from build123d import *

# Parameters (mm, degrees)
SKETCH1_W           = 100
SKETCH1_H           = 113.5
BOSS_EXTRUDE1_DEPTH = 8.5
CUT_EXTRUDE1_REACH  = 78.111
SKETCH2_W           = 83
SKETCH2_H           = 13.5
SKETCH2_H_2         = 13
SKETCH2_W_2         = 10
SKETCH2_H_3         = 10
SKETCH2_R           = 1.75
CUT_EXTRUDE2_REACH  = 78.111
SKETCH6_W           = 10
SKETCH6_H           = 10
CUT_EXTRUDE4_DEPTH  = 5.5
SKETCH7_R           = 3
SKETCH7_R_2         = 1.75
BOSS_EXTRUDE3_DEPTH = 5.5
FILLET1_R           = 1


with BuildPart() as part:
    # Sketch1 → Boss-Extrude1 (new body)
    with BuildSketch(Plane.XY):
        Rectangle(SKETCH1_W, SKETCH1_H)
    extrude(amount=BOSS_EXTRUDE1_DEPTH)

    # Sketch2 → Cut-Extrude1 (cut, up to next)
    with BuildSketch(Plane.XY.offset(8.5), mode=Mode.PRIVATE) as cut_extrude1_sk1:
        with Locations((0, 50)):
            Rectangle(SKETCH2_W, SKETCH2_H)
    cut_extrude1_tool1 = extrude(cut_extrude1_sk1.sketch, amount=-CUT_EXTRUDE1_REACH, mode=Mode.PRIVATE) & part.part
    # Sketch2 → Cut-Extrude1 (cut, up to next)
    with BuildSketch(Plane.XY.offset(8.5), mode=Mode.PRIVATE) as cut_extrude1_sk2:
        with BuildLine():
            ThreePointArc((-41.5, -29.75), (-39.156854249, -35.406854249), (-33.5, -37.75))
            Line((-33.5, -37.75), (33.5, -37.75))
            ThreePointArc((33.5, -37.75), (39.156854249, -35.406854249), (41.5, -29.75))
            Line((41.5, -29.75), (41.5, -0.25))
            Line((41.5, -0.25), (-41.5, -0.25))
            Line((-41.5, -0.25), (-41.5, -29.75))
        make_face()
    cut_extrude1_tool2 = extrude(cut_extrude1_sk2.sketch, amount=-CUT_EXTRUDE1_REACH, mode=Mode.PRIVATE) & part.part
    # Sketch2 → Cut-Extrude1 (cut, up to next)
    with BuildSketch(Plane.XY.offset(8.5), mode=Mode.PRIVATE) as cut_extrude1_sk3:
        with Locations((0, -50.25)):
            Rectangle(SKETCH2_W, SKETCH2_H_2)
    cut_extrude1_tool3 = extrude(cut_extrude1_sk3.sketch, amount=-CUT_EXTRUDE1_REACH, mode=Mode.PRIVATE) & part.part
    # Sketch2 → Cut-Extrude1 (cut, up to next)
    with BuildSketch(Plane.XY.offset(8.5), mode=Mode.PRIVATE) as cut_extrude1_sk4:
        with Locations((-11.75, 22.75)):
            Rectangle(SKETCH2_W_2, SKETCH2_H_3)
    cut_extrude1_tool4 = extrude(cut_extrude1_sk4.sketch, amount=-CUT_EXTRUDE1_REACH, mode=Mode.PRIVATE) & part.part
    # Sketch2 → Cut-Extrude1 (cut, up to next)
    with BuildSketch(Plane.XY.offset(8.5), mode=Mode.PRIVATE) as cut_extrude1_sk5:
        with Locations((45.75, 38.75)):
            Circle(SKETCH2_R)
    cut_extrude1_tool5 = extrude(cut_extrude1_sk5.sketch, amount=-CUT_EXTRUDE1_REACH, mode=Mode.PRIVATE) & part.part
    # Sketch2 → Cut-Extrude1 (cut, up to next)
    with BuildSketch(Plane.XY.offset(8.5), mode=Mode.PRIVATE) as cut_extrude1_sk6:
        with Locations((45.75, -38.75)):
            Circle(SKETCH2_R)
    cut_extrude1_tool6 = extrude(cut_extrude1_sk6.sketch, amount=-CUT_EXTRUDE1_REACH, mode=Mode.PRIVATE) & part.part
    # Sketch2 → Cut-Extrude1 (cut, up to next)
    with BuildSketch(Plane.XY.offset(8.5), mode=Mode.PRIVATE) as cut_extrude1_sk7:
        with Locations((-45.75, 38.75)):
            Circle(SKETCH2_R)
    cut_extrude1_tool7 = extrude(cut_extrude1_sk7.sketch, amount=-CUT_EXTRUDE1_REACH, mode=Mode.PRIVATE) & part.part
    # Sketch2 → Cut-Extrude1 (cut, up to next)
    with BuildSketch(Plane.XY.offset(8.5), mode=Mode.PRIVATE) as cut_extrude1_sk8:
        with Locations((-45.75, -38.75)):
            Circle(SKETCH2_R)
    cut_extrude1_tool8 = extrude(cut_extrude1_sk8.sketch, amount=-CUT_EXTRUDE1_REACH, mode=Mode.PRIVATE) & part.part
    add(cut_extrude1_tool1.solids().sort_by_distance((0, 50, 8.5))[0], mode=Mode.SUBTRACT)
    add(cut_extrude1_tool2.solids().sort_by_distance((0, -18.848961, 8.5))[0], mode=Mode.SUBTRACT)
    add(cut_extrude1_tool3.solids().sort_by_distance((0, -50.25, 8.5))[0], mode=Mode.SUBTRACT)
    add(cut_extrude1_tool4.solids().sort_by_distance((-11.75, 22.75, 8.5))[0], mode=Mode.SUBTRACT)
    add(cut_extrude1_tool5.solids().sort_by_distance((45.75, 38.75, 8.5))[0], mode=Mode.SUBTRACT)
    add(cut_extrude1_tool6.solids().sort_by_distance((45.75, -38.75, 8.5))[0], mode=Mode.SUBTRACT)
    add(cut_extrude1_tool7.solids().sort_by_distance((-45.75, 38.75, 8.5))[0], mode=Mode.SUBTRACT)
    add(cut_extrude1_tool8.solids().sort_by_distance((-45.75, -38.75, 8.5))[0], mode=Mode.SUBTRACT)

    # Sketch6 → Cut-Extrude2 (cut, up to next)
    with BuildSketch(Plane.XY.offset(8.5), mode=Mode.PRIVATE) as cut_extrude2_sk1:
        with BuildLine():
            Line((41.5, 8.25), (41.5, 29.25))
            ThreePointArc((41.5, 29.25), (39.156854249, 34.906854249), (33.5, 37.25))
            Line((33.5, 37.25), (28.5, 37.25))
            Line((28.5, 37.25), (28.5, 8.25))
            Line((28.5, 8.25), (33.5, 8.25))
            Line((33.5, 8.25), (41.5, 8.25))
        make_face()
    cut_extrude2_tool1 = extrude(cut_extrude2_sk1.sketch, amount=-CUT_EXTRUDE2_REACH, mode=Mode.PRIVATE) & part.part
    # Sketch6 → Cut-Extrude2 (cut, up to next)
    with BuildSketch(Plane.XY.offset(8.5), mode=Mode.PRIVATE) as cut_extrude2_sk2:
        with Locations((11.75, 22.75)):
            Rectangle(SKETCH6_W, SKETCH6_H)
    cut_extrude2_tool2 = extrude(cut_extrude2_sk2.sketch, amount=-CUT_EXTRUDE2_REACH, mode=Mode.PRIVATE) & part.part
    # Sketch6 → Cut-Extrude2 (cut, up to next)
    with BuildSketch(Plane.XY.offset(8.5), mode=Mode.PRIVATE) as cut_extrude2_sk3:
        with BuildLine():
            Line((-41.5, 8.25), (-41.5, 29.25))
            ThreePointArc((-41.5, 29.25), (-39.156854249, 34.906854249), (-33.5, 37.25))
            Line((-33.5, 37.25), (-28.5, 37.25))
            Line((-28.5, 37.25), (-28.5, 8.25))
            Line((-28.5, 8.25), (-33.5, 8.25))
            Line((-33.5, 8.25), (-41.5, 8.25))
        make_face()
    cut_extrude2_tool3 = extrude(cut_extrude2_sk3.sketch, amount=-CUT_EXTRUDE2_REACH, mode=Mode.PRIVATE) & part.part
    add(cut_extrude2_tool1.solids().sort_by_distance((34.821806, 22.269339, 8.5))[0], mode=Mode.SUBTRACT)
    add(cut_extrude2_tool2.solids().sort_by_distance((11.75, 22.75, 8.5))[0], mode=Mode.SUBTRACT)
    add(cut_extrude2_tool3.solids().sort_by_distance((-34.821806, 22.269339, 8.5))[0], mode=Mode.SUBTRACT)

    # Sketch8 → Cut-Extrude4 (cut)
    with BuildSketch(Plane.XY.offset(8.5)):
        with BuildLine():
            Line((-37.835, -40.7), (37.835, -40.7))
            ThreePointArc((37.835, -40.7), (38.836346779, -40.434383498), (39.567050808, -39.7))
            Line((39.567050808, -39.7), (40.811116722, -37.52))
            ThreePointArc((40.811116722, -37.52), (42.571113581, -35.629410248), (44.981116722, -34.7))
            ThreePointArc((44.981116722, -34.7), (46.210984272, -34.031299083), (46.701116722, -32.72))
            Line((46.701116722, -32.72), (46.701116722, 32.72))
            ThreePointArc((46.701116722, 32.72), (46.210984272, 34.031299083), (44.981116722, 34.7))
            ThreePointArc((44.981116722, 34.7), (42.571113581, 35.629410248), (40.811116722, 37.52))
            Line((40.811116722, 37.52), (39.567050808, 39.7))
            ThreePointArc((39.567050808, 39.7), (38.836346779, 40.434383498), (37.835, 40.7))
            Line((37.835, 40.7), (-37.835, 40.7))
            ThreePointArc((-37.835, 40.7), (-38.836346779, 40.434383498), (-39.567050808, 39.7))
            Line((-39.567050808, 39.7), (-40.811116722, 37.52))
            ThreePointArc((-40.811116722, 37.52), (-42.571113581, 35.629410248), (-44.981116722, 34.7))
            ThreePointArc((-44.981116722, 34.7), (-46.210984272, 34.031299083), (-46.701116722, 32.72))
            Line((-46.701116722, 32.72), (-46.701116722, -32.72))
            ThreePointArc((-46.701116722, -32.72), (-46.210984272, -34.031299083), (-44.981116722, -34.7))
            ThreePointArc((-44.981116722, -34.7), (-42.571113581, -35.629410248), (-40.811116722, -37.52))
            Line((-40.811116722, -37.52), (-39.567050808, -39.7))
            Line((-39.567050808, -39.7), (-37.835, -40.7))
        make_face()
    extrude(amount=-CUT_EXTRUDE4_DEPTH, mode=Mode.SUBTRACT)

    # Sketch7 → Boss-Extrude3 (add)
    # profile 1 of 8: a face of its own
    with BuildSketch(Plane.XY.offset(8.5)):
        with Locations((-24.25, 33.25)):
            Circle(SKETCH7_R)
        with Locations((-24.25, 33.25)):
            Circle(SKETCH7_R_2, mode=Mode.SUBTRACT)
    # profile 2 of 8: a face of its own
    with BuildSketch(Plane.XY.offset(8.5)):
        with Locations((-24.25, 12.25)):
            Circle(SKETCH7_R)
        with Locations((-24.25, 12.25)):
            Circle(SKETCH7_R_2, mode=Mode.SUBTRACT)
    # profile 3 of 8: a face of its own
    with BuildSketch(Plane.XY.offset(8.5)):
        with Locations((-11.75, 12.25)):
            Circle(SKETCH7_R)
        with Locations((-11.75, 12.25)):
            Circle(SKETCH7_R_2, mode=Mode.SUBTRACT)
    # profile 4 of 8: a face of its own
    with BuildSketch(Plane.XY.offset(8.5)):
        with Locations((11.75, 33.25)):
            Circle(SKETCH7_R)
        with Locations((11.75, 33.25)):
            Circle(SKETCH7_R_2, mode=Mode.SUBTRACT)
    # profile 5 of 8: a face of its own
    with BuildSketch(Plane.XY.offset(8.5)):
        with Locations((24.25, 33.25)):
            Circle(SKETCH7_R)
        with Locations((24.25, 33.25)):
            Circle(SKETCH7_R_2, mode=Mode.SUBTRACT)
    # profile 6 of 8: a face of its own
    with BuildSketch(Plane.XY.offset(8.5)):
        with Locations((11.75, 12.25)):
            Circle(SKETCH7_R)
        with Locations((11.75, 12.25)):
            Circle(SKETCH7_R_2, mode=Mode.SUBTRACT)
    # profile 7 of 8: a face of its own
    with BuildSketch(Plane.XY.offset(8.5)):
        with Locations((24.25, 12.25)):
            Circle(SKETCH7_R)
        with Locations((24.25, 12.25)):
            Circle(SKETCH7_R_2, mode=Mode.SUBTRACT)
    # profile 8 of 8: a face of its own
    with BuildSketch(Plane.XY.offset(8.5)):
        with Locations((-11.75, 33.25)):
            Circle(SKETCH7_R)
        with Locations((-11.75, 33.25)):
            Circle(SKETCH7_R_2, mode=Mode.SUBTRACT)
    extrude(amount=-BOSS_EXTRUDE3_DEPTH)

    # Fillet1
    fillet1_edges = [part.edges().sort_by_distance(p)[0] for p in [
        (45.75, -56.75, 0),
        (-45.75, 56.75, 0),
        (-45.75, -56.75, 8.5),
        (-45.75, 56.75, 8.5),
        (45.75, -56.75, 8.5),
        (-41.5, 56.75, 4.25),
        (41.5, 56.75, 4.25),
        (41.5, -56.75, 4.25),
        (-41.5, -56.75, 4.25),
        (-45.75, -56.75, 0),
        (45.75, 56.75, 0),
        (50, -56.75, 4.25),
        (-50, -56.75, 4.25),
        (-50, 56.75, 4.25),
        (50, 56.75, 4.25),
        (45.75, 56.75, 8.5),
    ]]
    fillet(fillet1_edges, radius=FILLET1_R)


solid = part.part
Geometry: final body of the model. Coordinates: model frame, mm. A direction names the side the tool comes from. Give positions to 0.01 mm unless a question says otherwise; leave off trailing zeros. Order: outer loops, then holes, each group sorted by start corner. A loop starts at its lowest first (then second) coordinate and runs counter-clockwise, first axis right, second up. Notation, with made-up numbers: (57, 82.25) -> (116, 82.25) arc R16 ccw to (116, 86.25) -> close; hole circle Ø9 at (69, -15.5). An arc over 180 degrees is marked (long way). Answer as a JSON object with one key per item and string values.
Q1. Section D-D (x = 20). Output: boundary loops of the cut face in (y, z).
Entries:
{"outline": "(-43.75, 0) -> (-37.75, 0) -> (-37.75, 3) -> (-40.7, 3) -> (-40.7, 8.5) -> (-43.75, 8.5) -> close; (-0.25, 0) -> (43.25, 0) -> (43.25, 8.5) -> (40.7, 8.5) -> (40.7, 3) -> (-0.25, 3) -> close"}
Q2. Draft query along X for faces 4 (the flat face through (-1, 13, 0)), 5 (the flat face through (-12, 27.75, 2)). Return one class per face: released by +X, released by -X, zero draft, split by the parting line, or undercut.
Entries:
{"face 4": "zero draft", "face 5": "undercut"}
Q3. Access query for faces 1 (the flat face through (-46.701, 0, 6)), 2 (the flat face through (41.5, 19, 2)), 3 (the flat face through (41.5, -50, 4)). Directions: +Z, -Z, +X, -X, +Y, -Y. A direction counts if a zero-diameter tool reaches every point of the face in a straight line with its end or side. Return the directions, or none.
Entries:
{"face 1": "+Z", "face 2": "+Z, -Z", "face 3": "+Z, -Z, -Y"}
Q4. Section A-A (x = -11.75). State how many separate pieces and enclosed holes the cut face has, plus the area to 3 significant figures.
Entries:
{"separate pieces": "3", "enclosed holes": "0", "area": "177 mm^2"}
Q5. First-contact query: pin 1 (1 mm diameter, centred on x = 11.5, y = 12.5, fed in from +Z); pin 2 (12 mm diameter, centred on x = 12, y = 37.5, fed in from +Z); pin 3 (4 mm diameter, centred on x = 16.5, z = 2.5, fed in from +Y); pin 4 (4 mm diameter, centred on x = -26, z = 6.5, fed in from -Y). Flat tips, straight axial feed; report the tip coordinate or a pass-through.
Entries:
{"pin 1": "stops at z = 3", "pin 2": "stops at z = 8.5", "pin 3": "stops at y = 43.25", "pin 4": "stops at y = -43.75"}
Q6. Section B-B (x = -24.25). Output: boundary loops of the cut face in (y, z).
Entries:
{"outline": "(-43.75, 0) -> (-37.75, 0) -> (-37.75, 3) -> (-40.7, 3) -> (-40.7, 8.5) -> (-43.75, 8.5) -> close; (-0.25, 0) -> (43.25, 0) -> (43.25, 8.5) -> (40.7, 8.5) -> (40.7, 3) -> (36.25, 3) -> (36.25, 8.5) -> (35, 8.5) -> (35, 3) -> (31.5, 3) -> (31.5, 8.5) -> (30.25, 8.5) -> (30.25, 3) -> (15.25, 3) -> (15.25, 8.5) -> (14, 8.5) -> (14, 3) -> (10.5, 3) -> (10.5, 8.5) -> (9.25, 8.5) -> (9.25, 3) -> (-0.25, 3) -> close"}
Q7. Material intervals for probe 1 along Y at (x, z) = (11.75, 5.05); probe 2 along Y at (x, z) = (-45.75, 2.5); probe 3 along X at (y, z) = (13, 2.5), sorted ascending.
Entries:
{"probe 1": "y = -43.75 to -40.7, 9.25 to 10.5, 14 to 15.25, 30.25 to 31.5, 35 to 36.25, 40.7 to 43.25", "probe 2": "y = -56.75 to -40.5, -37 to 37, 40.5 to 56.75", "probe 3": "x = -50 to -41.5, -28.5 to 28.5, 41.5 to 50"}
